```python
from build123d import *

# Parameters (mm, degrees)
SKETCH2_R               = 7.5
BOSS_EXTRUDE1_DEPTH     = 100
CUT_EXTRUDE1_DEPTH      = 101.560926806
CUT_EXTRUDE1_DEPTH_BACK = 101.560926806
SKETCH4_R               = 2.5
CUT_EXTRUDE2_DEPTH      = 10
SKETCH5_R               = 2.5
CUT_EXTRUDE3_DEPTH      = 5


with BuildPart() as part:
    # Sketch2 → Boss-Extrude1 (new body)
    with BuildSketch(Plane.XY):
        Circle(SKETCH2_R)
    extrude(amount=BOSS_EXTRUDE1_DEPTH)

    # Sketch3 → Cut-Extrude1 (cut, two sides: drawn at the far end of the back side and taken through both)
    with BuildSketch(Plane(origin=(0, 0, 0), x_dir=(0, 0, -1), z_dir=(1, 0, 0)).offset(-CUT_EXTRUDE1_DEPTH_BACK)):
        Polygon((-100, 7.5), (-86.572214113, -15.75760739), (-93.968196495, -20.02767981), (-105.531182824, 0), align=None)
        Polygon((0, 7.5), (-26.836822614, -7.99424676), (-23.788631199, -13.273869162), (1.512017142, -9.243577121), (5.324456029, -3.175017221), align=None)
    extrude(amount=CUT_EXTRUDE1_DEPTH + CUT_EXTRUDE1_DEPTH_BACK, mode=Mode.SUBTRACT)

    # Sketch4 → Cut-Extrude2 (cut)
    with BuildSketch(Plane(origin=(0, -41.426270189, 71.752404736), x_dir=(1, 0, 0), z_dir=(0, -0.5000000000000044, 0.866025403784436))):
        with Locations(Location((0, 47.834936491, 0), (0, 0, 270))):
            Circle(SKETCH4_R)
    extrude(amount=-CUT_EXTRUDE2_DEPTH, mode=Mode.SUBTRACT)

    # Sketch5 → Cut-Extrude3 (cut)
    with BuildSketch(Plane(origin=(0, 5.625, 3.247595264), x_dir=(1, 0, 0), z_dir=(0, -0.8660254037844386, -0.4999999999999999))):
        with Locations(Location((0, 11.25, 0), (0, 0, 270))):
            Circle(SKETCH5_R)
    extrude(amount=-CUT_EXTRUDE3_DEPTH, mode=Mode.SUBTRACT)


solid = part.part
```
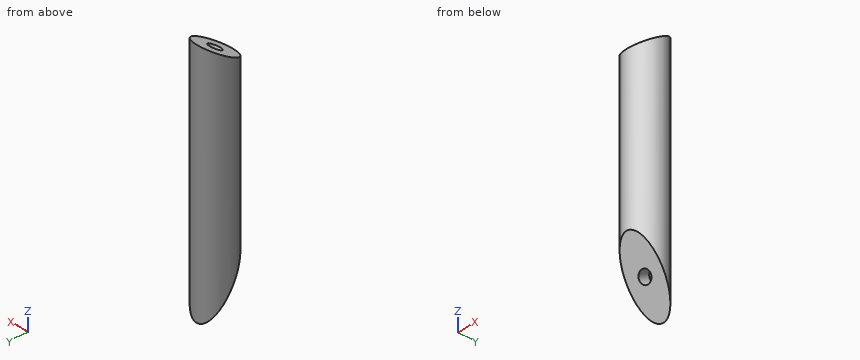
Read the model definition and answer for the solid it produces. Units are mm, in the model's axes. Give positions to 0.01 mm unless a question says otherwise; leave off trailing zeros. Order: outer loops, then holes, each group sorted by start corner. A loop starts at its lowest first (then second) coordinate and runs counter-clockwise, first axis right, second up.
(1) Straight lines are drawn through the part: L1, parallel to Z at x = 1, y = 3.5; L2, parallel to X at y = -0.5, z = 58. For each, find the intervals that lie inside material, in ascending order.
(2) Find section A-A (x = 0). Give the vertices of the cut face in (y, z), plus the area to 3 significant figures.
(3) Find section B-B (z = 45). Give the vertices of the cut face in (x, y), plus the area to 3 significant figures.
(4) Find section C-C (y = -4). Give the vertices of the cut face in (x, z), plus the area to 3 significant figures.
(5) Given pin 1 (1 mm diameter, centred on y = -2, z = 77.5, fed in from -X); pin 2 (1 mm diameter, centred on x = 1.5, z = 70, fed in from -Y); pin 3 (2 mm diameter, centred on y = -4.5, z = 22.5, fed in from -X), each flat-ended and moving along its own axis, determine where each tip first touches the part or whether it passes through.
(6) Find section D-D (y = 4.5). Give the number of separate pieces and of enclosed holes in the cut face, plus the area to 3 significant figures.
Result sheet:
1. L1: z = 6.93 to 12.37, 16.93 to 86.14, 94.19 to 97.69
1. L2: x = -7.48 to 7.48
2. outline: (-7.5, 25.98) - (-1.25, 15.16) - (3.08, 17.66) - (5.58, 13.33) - (1.25, 10.83) - (7.5, 0) - (7.5, 100) - (2.17, 96.92) - (7.17, 88.26) - (2.83, 85.76) - (-2.17, 94.42) - (-7.5, 91.34) - close
2. area: 1,170 mm2
3. outline: circle Ø15 at (0, 0)
3. area: 177 mm2
4. outline: (-6.34, 19.92) - (6.34, 19.92) - (6.34, 93.36) - (-6.34, 93.36) - close
4. area: 932 mm2
5. pin 1: stops at x = -7.35
5. pin 2: stops at y = -7.43
5. pin 3: stops at x = -6.63
6. separate pieces: 1
6. enclosed holes: 2
6. area: 1,080 mm2
